Model file for the job. Use its own axes, mm. Face numbers are marked on the shaded views. A direction names the side the tool comes from. Give positions to 0.01 mm unless a question says otherwise; leave off trailing zeros. Order: outer loops, then holes, each group sorted by start corner. A loop starts at its lowest first (then second) coordinate and runs counter-clockwise, first axis right, second up. Notation, with made-up numbers: M 84,9.25 L 137,9.25 A21 cw 137,33.25 Z; hole C 13.5,3.25 d1. An arc over 180 degrees is marked long. Return JSON: item names as keys, results as strings. Group by question number.
1. Slice it at D-D on x = 40. List the corners of the cut face in (y, z).
2. Wall check: probe 1 along Z at (x, y) = (38.65, 49); probe 2 along Z at (x, y) = (41, 36); probe 3 along X at (y, z) = (36, -9.5). Give the ranges that are in metal, low to high. Write a range as [from, to].
3. 3-axis set-ups, long thin cutter, end or side, ignore diameter. For the marked faces 4, 5 and 6: which of +Z, -Z, +X, -X, +Y, -Y reach the whole face in a straight line?
4. Two-plate mould, pull along Z, no slides. Class the marked faces 1, 2 and 3: released by +Z, released by -Z, zero draft, split by the parting line, or undercut.
5. Slice it at C-C on y = 31. List the corners of the cut face in (x, z).
6. Pin check, flat tips, straight feed: pin 1 (1.2 mm diameter, centred on x = 35, y = 59, fed in from -Z); pin 2 (3 mm diameter, centred on x = 30.5, z = -11, fed in from -Y); pin 3 (4 mm diameter, centred on x = 26, z = -54, fed in from +Y); pin 4 (3 mm diameter, centred on y = 60.5, z = -26.5, fed in from -X). Stop position of each tip, or through.
7. Slice it at A-A on x = 21. List the corners of the cut face in (y, z) (3 decimals), then the cut area to 4 significant figures.
8. Slice it at B-B on z = -48. List the corners of the cut face in (x, y).
from build123d import *

# Parameters (mm, degrees)
SKETCH_1_W           = 45
SKETCH_1_H           = 42
EXTRUDE_1_DEPTH      = 5
SKETCH_3_R           = 14.775
SKETCH_3_R_2         = 2
CUT_EXTRUDE_1_DEPTH  = 13
SKETCH_7_W           = 18
SKETCH_7_H           = 5
EXTRUDE_3_DEPTH      = 10
SKETCH_8_W           = 18
SKETCH_8_H           = 5
EXTRUDE_4_DEPTH      = 10
EXTRUDE_5_DEPTH      = 53
EXTRUDE_6_DEPTH      = 15
EXTRUDE_6_DEPTH_BACK = 77
SKETCH_11_W          = 18
SKETCH_11_H          = 7
SKETCH_12_W          = 57
SKETCH_12_H          = 14
CUT_EXTRUDE_2_DEPTH  = 10
SKETCH_15_R          = 2.25
CUT_EXTRUDE_5_DEPTH  = 10
SKETCH_16_W          = 6
SKETCH_16_H          = 62
EXTRUDE_7_DEPTH      = 4
SKETCH_17_W          = 5
SKETCH_17_H          = 9.7027375
EXTRUDE_8_DEPTH      = 42
SKETCH_13_R          = 2
CUT_EXTRUDE_3_DEPTH  = 16
CUT_EXTRUDE_4_DEPTH  = 3
FILLET_1_R           = 4
FILLET_2_R           = 2


with BuildPart() as part:
    # Эскиз1 → Бобышка-Вытянуть1 (new body)
    with BuildSketch(Plane(origin=(0, 0, 0), x_dir=(1, 0, 0), z_dir=(0, 1, 0))):
        with Locations((22.5, 21)):
            Rectangle(SKETCH_1_W, SKETCH_1_H)
    extrude(amount=EXTRUDE_1_DEPTH)

    # Эскиз3 → Вырез-Вытянуть1 (cut)
    with BuildSketch(Plane.XZ):
        with Locations(Location((21, -21, 0), (0, 0, 270))):
            Circle(SKETCH_3_R)
        with Locations(Location((36.5, -5.5, 0), (0, 0, 270))):
            Circle(SKETCH_3_R_2)
        with Locations(Location((5.5, -5.5, 0), (0, 0, 270))):
            Circle(SKETCH_3_R_2)
        with Locations(Location((5.5, -36.5, 0), (0, 0, 270))):
            Circle(SKETCH_3_R_2)
        with Locations(Location((36.5, -36.5, 0), (0, 0, 270))):
            Circle(SKETCH_3_R_2)
    extrude(amount=-CUT_EXTRUDE_1_DEPTH, mode=Mode.SUBTRACT)

    # Эскиз7 → Бобышка-Вытянуть3 (add)
    with BuildSketch(Plane.XY):
        with Locations((36, 2.5)):
            Rectangle(SKETCH_7_W, SKETCH_7_H)
    extrude(amount=EXTRUDE_3_DEPTH)

    # Эскиз8 → Бобышка-Вытянуть4 (add)
    with BuildSketch(Plane(origin=(0, 0, -42), x_dir=(-1, 0, 0), z_dir=(0, 0, -1))):
        with Locations((-36, 2.5)):
            Rectangle(SKETCH_8_W, SKETCH_8_H)
    extrude(amount=EXTRUDE_4_DEPTH)

    # Эскиз10 → Бобышка-Вытянуть5 (add)
    with BuildSketch(Plane(origin=(0, 5, 0), x_dir=(1, 0, 0), z_dir=(0, 1, 0))):
        Polygon((27, 52), (45, 52), (45, -10), (27, -10), (27, 0), (42, 0), (42, 42), (27, 42), align=None)
    extrude(amount=EXTRUDE_5_DEPTH)

    # Эскиз11 → Бобышка-Вытянуть6 (add, two sides: drawn at the far end of the back side and taken through both)
    with BuildSketch(Plane(origin=(0, 0, -52), x_dir=(-1, 0, 0), z_dir=(0, 0, -1)).offset(-EXTRUDE_6_DEPTH_BACK)):
        with Locations((-36, 54.5)):
            Rectangle(SKETCH_11_W, SKETCH_11_H)
    extrude(amount=EXTRUDE_6_DEPTH + EXTRUDE_6_DEPTH_BACK)

    # Эскиз12 → Вырез-Вытянуть2 (cut)
    with BuildSketch(Plane.ZY.offset(-27)):
        with Locations((-21, 49)):
            Rectangle(SKETCH_12_W, SKETCH_12_H)
    extrude(amount=-CUT_EXTRUDE_2_DEPTH, mode=Mode.SUBTRACT)

    # Эскиз15 → Вырез-Вытянуть5 (cut)
    with BuildSketch(Plane(origin=(0, 58, 0), x_dir=(1, 0, 0), z_dir=(0, 1, 0))):
        with Locations(Location((36, -17, 0), (0, 0, 270))):
            Circle(SKETCH_15_R)
        with Locations(Location((36, 59, 0), (0, 0, 270))):
            Circle(SKETCH_15_R)
    extrude(amount=-CUT_EXTRUDE_5_DEPTH, mode=Mode.SUBTRACT)

    # Эскиз16 → Бобышка-Вытянуть7 (add)
    with BuildSketch(Plane(origin=(0, 58, 0), x_dir=(1, 0, 0), z_dir=(0, 1, 0))):
        with Locations((36, 21)):
            Rectangle(SKETCH_16_W, SKETCH_16_H)
    extrude(amount=EXTRUDE_7_DEPTH)

    # Эскиз17 → Бобышка-Вытянуть8 (add)
    with BuildSketch(Plane.XY.offset(-42)):
        with Locations((39.5, 46.85136875)):
            Rectangle(SKETCH_17_W, SKETCH_17_H)
    extrude(amount=EXTRUDE_8_DEPTH)

    # Эскиз13 → Вырез-Вытянуть3 (cut)
    with BuildSketch(Plane.ZY.offset(-45)):
        with Locations((-42, 49)):
            Circle(SKETCH_13_R)
        with Locations((0, 49)):
            Circle(SKETCH_13_R)
    extrude(amount=CUT_EXTRUDE_3_DEPTH, mode=Mode.SUBTRACT)

    # Эскиз14 → Вырез-Вытянуть4 (cut)
    with BuildSketch(Plane(origin=(45, 0, 0), x_dir=(0, 0, -1), z_dir=(1, 0, 0))):
        Polygon((2.165063509, 52.75), (-2.165063509, 52.75), (-4.330127019, 49), (-2.165063509, 45.25), (2.165063509, 45.25), (4.330127019, 49), align=None)
        Polygon((44.165063509, 52.75), (39.834936491, 52.75), (37.669872981, 49), (39.834936491, 45.25), (44.165063509, 45.25), (46.330127019, 49), align=None)
    extrude(amount=-CUT_EXTRUDE_4_DEPTH, mode=Mode.SUBTRACT)

    # Скругление1
    fillet_1_edges = [part.edges().sort_by_distance(p)[0] for p in [
        (27, 23.5, 0),
        (27, 23.5, -42),
        (0, 2.5, -42),
        (0, 2.5, 0),
        (45, 54.5, 25),
        (27, 54.5, 25),
        (45, 54.5, -67),
        (27, 54.5, -67),
    ]]
    fillet(fillet_1_edges, radius=FILLET_1_R)

    # Скругление2
    fillet_2_edges = [part.edges().sort_by_distance(p)[0] for p in [
        (45, 25.5, 10),
        (27, 25.5, -52),
        (45, 25.5, -52),
        (27, 25.5, 10),
    ]]
    fillet(fillet_2_edges, radius=FILLET_2_R)


solid = part.part
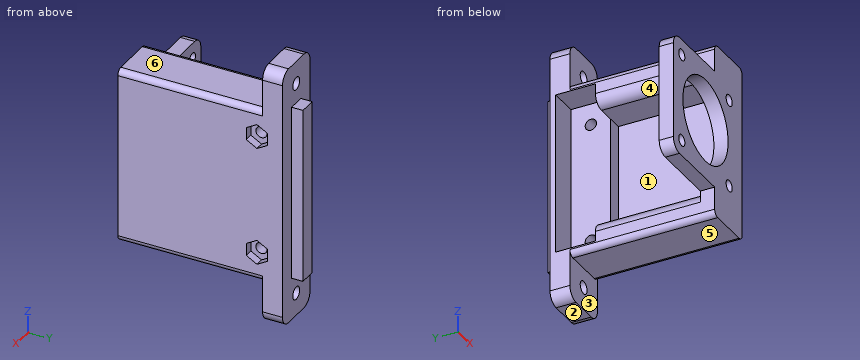
Result:
{
 "1": {"outline": "M 0,-52 L 51,-52 L 51,-67 L 58,-67 L 58,25 L 51,25 L 51,10 L 0,10 Z; hole M 5,-42 L 42,-42 L 42,0 L 5,0 Z; hole C 49,-42 d4; hole C 49,0 d4"},
 "2": {"probe 1": "z = [-52, -44], [-40, -2], [2, 10]", "probe 2": "z = [-52, -42], [0, 10]", "probe 3": "x = [42, 45]"},
 "3": {"face 4": "-X", "face 5": "-Z, +X, -X, -Y", "face 6": "+Z, +X, -X, -Y"},
 "4": {"face 1": "undercut", "face 2": "released by -Z", "face 3": "zero draft"},
 "5": {"outline": "M 27,-50 A2 ccw 29,-52 L 43,-52 A2 ccw 45,-50 L 45,8 A2 ccw 43,10 L 29,10 A2 ccw 27,8 L 27,4 A4 ccw 31,0 L 42,0 L 42,-42 L 31,-42 A4 ccw 27,-46 Z"},
 "6": {"pin 1": "stops at z = -52", "pin 2": "stops at y = 0", "pin 3": "stops at y = 58", "pin 4": "stops at x = 33"},
 "7": {"outline": "M 0,-42 L 5,-42 L 5,-35.775 L 0,-35.775 Z; M 0,-6.225 L 5,-6.225 L 5,0 L 0,0 Z", "area": "62.25 mm2"},
 "8": {"outline": "M 27,0 L 45,0 L 45,58 L 39,58 L 39,62 L 33,62 L 33,58 L 27,58 L 27,56 L 37,56 L 37,42 L 27,42 Z"}
}
